The listing builds one solid part. Answer for the finished solid, in the listing's coordinates (mm). Face numbers are marked on the shaded views. Round coordinates to 2 decimals unless told otherwise and drop trailing zeros. Write each loop counter-clockwise with the first axis right and the second up, starting at its lowest first coordinate (ties: lowest second). Pieces come first, ordered by that corner, then holes.
(1) A cutting plane is placed at C-C, the plane x = -31.5. Give the vertices of the cut face in (y, z), and give its area (3 significant figures).
(2) A cutting plane is placed at A-A, the plane z = 2.25. Give the number of separate pieces and of enclosed holes in the cut face, and give its area (3 significant figures).
(3) The mould has two halves that part along Y. Classify the marked faces 1 and 2: +Y half, -Y half, draft (parallel to the pull), parting line (faces both ways), or undercut.
(4) A cutting plane is placed at D-D, the plane y = -397. Give the vertices of the cut face in (x, z).
(5) A cutting plane is placed at B-B, the plane y = 150. Give the vertices of the cut face in (x, z), and give its area (3 significant figures).
(6) Each of these flat-tipped pins is pushed along its axis until it touches: pin 1 Ø1.6 at (x, z) = (-64.5, 6) entering from +Y; pin 2 Ø0.6 at (y, z) = (207.5, 5.5) entering from -X; pin 3 Ø0.6 at (y, z) = (86.5, 6.5) entering from -X; pin 4 Ø7 at (x, y) = (217.5, 125) entering from +Z. Where does it stop, or does it pass through?
(7) Find the intervals of material crossed by probe 1 along Y at (x, z) = (135, 5.25); probe 2 along X at (y, z) = (141, 0.5); probe 3 along Y at (x, z) = (217.5, 1.55), in increasing order.
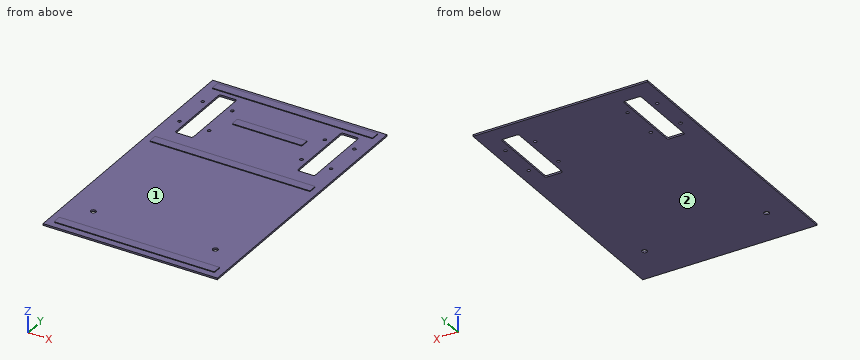
from build123d import *

# Parameters (mm, degrees)
F0_W     = 500
F0_H     = 800
F0_R     = 7.5
F0_R_2   = 4.5
F1_DEPTH = 5
F3_DEPTH = 2


with BuildPart() as f1:
    # F0 (on Top) → F1 (new body)
    with BuildSketch(Plane.XY):
        with Locations((0, -175)):
            Rectangle(F0_W, F0_H)
        with Locations((-175, -461)):
            Circle(F0_R, mode=Mode.SUBTRACT)
        with Locations((175, -461)):
            Circle(F0_R, mode=Mode.SUBTRACT)
        with Locations((-217.5, 15)):
            Circle(F0_R_2, mode=Mode.SUBTRACT)
        with Locations((-132.5, 15)):
            Circle(F0_R_2, mode=Mode.SUBTRACT)
        with BuildLine():
            ThreePointArc((-200, 170), (-198.535534, 173.535534), (-195, 175))
            Line((-195, 175), (-155, 175))
            ThreePointArc((-155, 175), (-151.464466, 173.535534), (-150, 170))
            Line((-150, 170), (-150, -30))
            ThreePointArc((-150, -30), (-151.464466, -33.535534), (-155, -35))
            Line((-155, -35), (-195, -35))
            ThreePointArc((-195, -35), (-198.535534, -33.535534), (-200, -30))
            Line((-200, -30), (-200, 170))
        make_face(mode=Mode.SUBTRACT)
        with Locations((-217.5, 125)):
            Circle(F0_R_2, mode=Mode.SUBTRACT)
        with Locations((-132.5, 125)):
            Circle(F0_R_2, mode=Mode.SUBTRACT)
        with Locations((132.5, 15)):
            Circle(F0_R_2, mode=Mode.SUBTRACT)
        with Locations((217.5, 15)):
            Circle(F0_R_2, mode=Mode.SUBTRACT)
        with BuildLine():
            Line((195, -35), (155, -35))
            ThreePointArc((155, -35), (151.464466, -33.535534), (150, -30))
            Line((150, -30), (150, 170))
            ThreePointArc((150, 170), (151.464466, 173.535534), (155, 175))
            Line((155, 175), (195, 175))
            ThreePointArc((195, 175), (198.535534, 173.535534), (200, 170))
            Line((200, 170), (200, -30))
            ThreePointArc((200, -30), (198.535534, -33.535534), (195, -35))
        make_face(mode=Mode.SUBTRACT)
        with Locations((132.5, 125)):
            Circle(F0_R_2, mode=Mode.SUBTRACT)
        with Locations((217.5, 125)):
            Circle(F0_R_2, mode=Mode.SUBTRACT)
    extrude(amount=F1_DEPTH)

    # F2 (on face) → F3 (join)
    with BuildSketch(Plane.XY.offset(5)):
        with BuildLine():
            Line((228, 215), (-228, 215))
            ThreePointArc((-228, 215), (-229.414214, 214.414214), (-230, 213))
            Line((-230, 213), (-230, 192))
            ThreePointArc((-230, 192), (-229.414214, 190.585786), (-228, 190))
            Line((-228, 190), (228, 190))
            ThreePointArc((228, 190), (229.414214, 190.585786), (230, 192))
            Line((230, 192), (230, 213))
            ThreePointArc((230, 213), (229.414214, 214.414214), (228, 215))
        make_face()
        with BuildLine():
            Line((98, 95), (-98, 95))
            ThreePointArc((-98, 95), (-99.414214, 94.414214), (-100, 93))
            Line((-100, 93), (-100, 72))
            ThreePointArc((-100, 72), (-99.414214, 70.585786), (-98, 70))
            Line((-98, 70), (98, 70))
            ThreePointArc((98, 70), (99.414214, 70.585786), (100, 72))
            Line((100, 72), (100, 93))
            ThreePointArc((100, 93), (99.414214, 94.414214), (98, 95))
        make_face()
        with BuildLine():
            Line((228, -79.874295), (-228, -79.874295))
            ThreePointArc((-228, -79.874295), (-229.414214, -80.460082), (-230, -81.874295))
            Line((-230, -81.874295), (-230, -102.874295))
            ThreePointArc((-230, -102.874295), (-229.414214, -104.288509), (-228, -104.874295))
            Line((-228, -104.874295), (228, -104.874295))
            ThreePointArc((228, -104.874295), (229.414214, -104.288509), (230, -102.874295))
            Line((230, -102.874295), (230, -81.874295))
            ThreePointArc((230, -81.874295), (229.414214, -80.460082), (228, -79.874295))
        make_face()
        with BuildLine():
            Line((228, -531.046275), (-228, -531.046275))
            ThreePointArc((-228, -531.046275), (-229.414214, -531.632061), (-230, -533.046275))
            Line((-230, -533.046275), (-230, -554.046275))
            ThreePointArc((-230, -554.046275), (-229.414214, -555.460488), (-228, -556.046275))
            Line((-228, -556.046275), (228, -556.046275))
            ThreePointArc((228, -556.046275), (229.414214, -555.460488), (230, -554.046275))
            Line((230, -554.046275), (230, -533.046275))
            ThreePointArc((230, -533.046275), (229.414214, -531.632061), (228, -531.046275))
        make_face()
    extrude(amount=F3_DEPTH)


solid = f1.part
Solutions:
1. outline: (-575, 0) - (225, 0) - (225, 5) - (215, 5) - (215, 7) - (190, 7) - (190, 5) - (95, 5) - (95, 7) - (70, 7) - (70, 5) - (-79.87, 5) - (-79.87, 7) - (-104.87, 7) - (-104.87, 5) - (-531.05, 5) - (-531.05, 7) - (-556.05, 7) - (-556.05, 5) - (-575, 5) - close
1. area: 4,200 mm2
2. separate pieces: 1
2. enclosed holes: 12
2. area: 378,000 mm2
3. face 1: undercut
3. face 2: draft
4. outline: (-250, 0) - (250, 0) - (250, 5) - (-250, 5) - close
5. outline: (-250, 0) - (-200, 0) - (-200, 5) - (-250, 5) - close; (-150, 0) - (150, 0) - (150, 5) - (-150, 5) - close; (200, 0) - (250, 0) - (250, 5) - (200, 5) - close
5. area: 2,000 mm2
6. pin 1: stops at y = 215
6. pin 2: stops at x = -230
6. pin 3: stops at x = -100
6. pin 4: passes through
7. probe 1: y = -556.05 to -531.05, -104.87 to -79.87, 190 to 215
7. probe 2: x = -250 to -200, -150 to 150, 200 to 250
7. probe 3: y = -575 to 10.5, 19.5 to 120.5, 129.5 to 225
